Can you work these out from the model? Positions are in its coordinate system, mm. Coordinates: 2 decimals unless noted, no trailing zeros. Loops run counter-clockwise (first coordinate to the right, second up) from the corner with the lowest first, then second, coordinate; pieces in that order, holes last.
```python
from build123d import *

# Parameters (mm, degrees)
CROQUIS1_R              = 2.5
CROQUIS1_R_2            = 2
SALIENTE_EXTRUIR2_DEPTH = 20
REDONDEO5_R             = 0.1
REDONDEO6_R             = 0.2


with BuildPart() as part:
    # Croquis1 → Saliente-Extruir2 (new body)
    with BuildSketch(Plane.XY):
        Circle(CROQUIS1_R)
        Circle(CROQUIS1_R_2, mode=Mode.SUBTRACT)
    extrude(amount=SALIENTE_EXTRUIR2_DEPTH)

    # Redondeo5
    redondeo5_edges = [part.edges().sort_by_distance(p)[0] for p in [
        (-2.5, 0, 0),
        (-2.5, 0, 20),
    ]]
    fillet(redondeo5_edges, radius=REDONDEO5_R)

    # Redondeo6
    redondeo6_edges = [part.edges().sort_by_distance(p)[0] for p in [
        (-2, 0, 0),
        (-2, 0, 20),
    ]]
    fillet(redondeo6_edges, radius=REDONDEO6_R)


solid = part.part
```
Item 1: I'm going to push a flat-ended pin straight in: P1, Ø1.5, axis at y = 1.5, z = 7, coming from the -X side. Where does the tip first touch, or does it pass through?
Results are:
P1: stops at x = -2.38
Item 2: Suppose I cut it at A-A, the plane x = 0. Please give me the cut outline in (y, z), plus the area to 3 significant figures.
Results are:
outline: (-2.5, 0.1) arc R0.1 ccw to (-2.4, 0) - (-2.2, 0) arc R0.2 ccw to (-2, 0.2) - (-2, 19.8) arc R0.2 ccw to (-2.2, 20) - (-2.4, 20) arc R0.1 ccw to (-2.5, 19.9) - close; (2, 0.2) arc R0.2 ccw to (2.2, 0) - (2.4, 0) arc R0.1 ccw to (2.5, 0.1) - (2.5, 19.9) arc R0.1 ccw to (2.4, 20) - (2.2, 20) arc R0.2 ccw to (2, 19.8) - close
area: 20.0 mm2
Item 3: Suppose I cut it at C-C, the plane z = 11.25. Please give me the cut outline in (x, y), plus the area to 3 significant figures.
Results are:
outline: circle Ø5 at (0, 0); hole circle Ø4 at (0, 0)
area: 7.07 mm2
Item 4: I need wall thicknesses on line 1 along Y through (x, z) = (0, 11.5); line 2 along X through (y, z) = (1.65, 8.5). Which ranges of each line are inside material? Lowest first, please.
Results are:
line 1: y = -2.5 to -2, 2 to 2.5
line 2: x = -1.88 to -1.13, 1.13 to 1.88
Item 5: We'd pull the mould along X, two halves only. Please class faces 1 (the face through (0, -2, 10)), 2 (the face through (-0.54, -2.44, 9.86)): +X half, -X half, draft (parallel to the pull), parting line (faces both ways), or undercut.
Results are:
face 1: undercut
face 2: parting line
